```python
from build123d import *

# Parameters (mm, degrees)
BOSS_EXTRUDE1_DEPTH = 5
CUT_EXTRUDE6_DEPTH  = 32.7
CUT_EXTRUDE7_DEPTH  = 32.7
CUT_EXTRUDE8_DEPTH  = 50
SKETCH10_W          = 10
SKETCH10_H          = 4
CUT_EXTRUDE9_DEPTH  = 6


with BuildPart() as part:
    # Sketch1 → Boss-Extrude1 (new body)
    with BuildSketch(Plane.XY):
        Polygon((0, 0), (240, 0), (240, 72.25), (225, 72.25), (225, 70.25), (210, 70.25), (210, 54), (210, 50), (30, 50), (30, 54), (20, 54), (20, 70.25), (15, 70.25), (15, 72.25), (0, 72.25), align=None)
    extrude(amount=BOSS_EXTRUDE1_DEPTH)

    # Sketch7 → Cut-Extrude6 (cut)
    with BuildSketch(Plane(origin=(76.962340789, 50, 79.982193432), x_dir=(0.299340075, 0, -0.954146488), z_dir=(0, -1, 0))):
        Polygon((89.56567359, 88.367941315), (121.015834787, 78.501224076), (119.481716905, 73.611223328), (88.031555708, 83.477940566), align=None)
    extrude(amount=CUT_EXTRUDE6_DEPTH, mode=Mode.SUBTRACT)

    # Sketch8 → Cut-Extrude7 (cut)
    with BuildSketch(Plane(origin=(151.064056229, 50, -36.816333928), x_dir=(-0.299340075, 0, 0.954146488), z_dir=(0, -1, 0))):
        Polygon((48.269879058, 101.323484697), (121.015834787, 78.501224076), (119.481716905, 73.611223328), (46.735761176, 96.433483948), align=None)
    extrude(amount=CUT_EXTRUDE7_DEPTH, mode=Mode.SUBTRACT)

    # Sketch9 → Cut-Extrude8 (cut)
    with BuildSketch(Plane(origin=(179.822929518, 98.166866164, 0), x_dir=(-1, 0, 0), z_dir=(0, 0, -1))):
        Polygon((91.809731009, -83.166866164), (73.384731009, -83.166866164), (73.384731009, -88.166866164), (58.234731009, -88.166866164), (58.234731009, -83.166866164), (39.809731009, -83.166866164), (39.809731009, -75.166866164), (91.809731009, -75.166866164), align=None)
    extrude(amount=-CUT_EXTRUDE8_DEPTH, mode=Mode.SUBTRACT)

    # Sketch10 → Cut-Extrude9 (cut, through all)
    with BuildSketch(Plane.XY.offset(5)):
        with Locations((20, 2)):
            Rectangle(SKETCH10_W, SKETCH10_H)
        with Locations((220, 2)):
            Rectangle(SKETCH10_W, SKETCH10_H)
    extrude(amount=-CUT_EXTRUDE9_DEPTH, mode=Mode.SUBTRACT)


solid = part.part
```
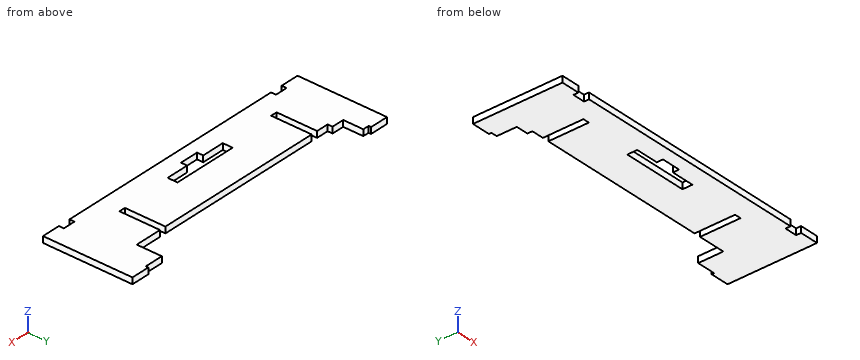
Geometry check sheet. Reference: the model listing, model coordinates, mm. Give positions to 0.01 mm unless a question says otherwise; leave off trailing zeros. Order: outer loops, then holes, each group sorted by start corner. A loop starts at its lowest first (then second) coordinate and runs counter-clockwise, first axis right, second up.
1. Thickness scan on L1, parallel to X at y = 33, z = 3; L2, parallel to X at y = 21.5, z = 3.9; L3, parallel to X at y = 60, z = 3.05. Record the ranges inside material, lowest first.
2. Section check D-D, the plane x = 144. Enter the section's corners in (y, z).
3. Section check C-C, the plane y = 64.5. Enter the section's corners in (x, z), and give its area (3 significant figures).
4. Section check A-A, the plane x = 118.5. Enter the section's corners in (y, z).
5. Section check B-B, the plane y = 34. Enter the section's corners in (x, z).
6. Gauge pin test, flat ends, axial feed: pin 1 Ø3 at (y, z) = (1.5, 2.5) entering from -X; pin 2 Ø2.5 at (x, z) = (17, 3) entering from +Y; pin 3 Ø1.5 at (x, z) = (136, 3) entering from +Y; pin 4 Ø2.5 at (x, z) = (220.5, 1.5) entering from -Y. Record the tip position at first contact, or that the pin passes through.
Values follow:
1. L1: x = 0 to 39.94, 45.06 to 182.96, 188.09 to 240
1. L2: x = 0 to 39.94, 45.06 to 88.01, 140.01 to 182.96, 188.09 to 240
1. L3: x = 0 to 20, 210 to 240
2. outline: (0, 0) - (50, 0) - (50, 5) - (0, 5) - close
3. outline: (0, 0) - (20, 0) - (20, 5) - (0, 5) - close; (210, 0) - (240, 0) - (240, 5) - (210, 5) - close
3. area: 250 mm2
4. outline: (0, 0) - (10, 0) - (10, 5) - (0, 5) - close; (23, 0) - (50, 0) - (50, 5) - (23, 5) - close
5. outline: (0, 0) - (39.94, 0) - (39.94, 5) - (0, 5) - close; (45.06, 0) - (182.96, 0) - (182.96, 5) - (45.06, 5) - close; (188.09, 0) - (240, 0) - (240, 5) - (188.09, 5) - close
6. pin 1: stops at x = 0
6. pin 2: stops at y = 70.25
6. pin 3: stops at y = 50
6. pin 4: stops at y = 4
